Autodesk Inventor part; units mm, degrees
ref_plane "YZ Plane" through (0, 0, 0) normal (1, 0, 0) x (0, 1, 0)
ref_plane "XZ Plane" through (0, 0, 0) normal (0, 1, 0) x (-1, 0, 0)
ref_plane "XY Plane" through (0, 0, 0) normal (0, 0, 1) x (1, 0, 0)
sketch "Sketch1" plane through (0, 0, 0) normal (0, 1, 0) x (-1, 0, 0)
  line L0 (0, 0) -> (50, 0)
  line L1 (50, 0) -> (50, 48)
  line L2 (50, 48) -> (0, 48)
  line L3 (0, 48) -> (0, 0)
  dimension "d0" = 50
  dimension "d1" = 48
extrude "Extrusion1" add sketch "Sketch1" along normal blind 1.8
sketch "Sketch4" plane through (0, 1.8, 0) normal (0, 1, 0) x (1, 0, 0)
  line L0 (0, 0) -> (-50, 0)
  line L1 (-50, 0) -> (-50, -48)
  line L2 (-48, -17.9) -> (-40, -17.9)
  line L3 (-40, -17.9) -> (-40, -31.1)
  line L4 (-40, -31.1) -> (-48, -31.1)
  line L5 (-48, -31.1) -> (-48, -17.9)
  line L6 (-44, -24.5) -> (-44, -17.9)
  line L7 (-44, -24.5) -> (-40, -24.5)
  line L8 (-44, -24.5) -> (-44, -31.1)
  line L9 (-44, -24.5) -> (-48, -24.5)
  line L10 (-39, -17.9) -> (-31, -17.9)
  line L11 (-31, -17.9) -> (-31, -31.1)
  line L12 (-31, -31.1) -> (-39, -31.1)
  line L13 (-39, -31.1) -> (-39, -17.9)
  line L14 (-35, -24.5) -> (-35, -17.9)
  line L15 (-35, -24.5) -> (-31, -24.5)
  line L16 (-35, -24.5) -> (-35, -31.1)
  line L17 (-35, -24.5) -> (-39, -24.5)
  line L18 (-19, -17.9) -> (-11, -17.9)
  line L19 (-11, -17.9) -> (-11, -31.1)
  line L20 (-11, -31.1) -> (-19, -31.1)
  line L21 (-19, -31.1) -> (-19, -17.9)
  line L22 (-15, -24.5) -> (-15, -17.9)
  line L23 (-15, -24.5) -> (-11, -24.5)
  line L24 (-15, -24.5) -> (-15, -31.1)
  line L25 (-15, -24.5) -> (-19, -24.5)
  line L26 (-2, -17.9) -> (-2, -31.1)
  line L27 (-6, -24.5) -> (-6, -17.9)
  line L28 (-6, -24.5) -> (-2, -24.5)
  line L29 (-6, -24.5) -> (-6, -31.1)
  line L30 (-2, -31.1) -> (-10, -31.1)
  line L31 (-10, -17.9) -> (-2, -17.9)
  line L32 (-6, -24.5) -> (-10, -24.5)
  line L33 (-10, -31.1) -> (-10, -17.9)
  dimension "d4" = 8
  dimension "d6" = 13.2
  dimension "d7" = 24.5
  dimension "d8" = 6
  dimension "d9" = 8
  dimension "d10" = 13.2
  dimension "d12" = 9
  dimension "d13" = 8
  dimension "d14" = 13.2
  dimension "d15" = 8
  dimension "d16" = 13.2
  dimension "d17" = 20
  dimension "d18" = 9
extrude "Extrusion2" add sketch "Sketch4" along normal blind 10
sketch "Sketch5" plane through (0, 11.8, 0) normal (0, 1, 0) x (1, 0, 0)
  line L0 (-31, -31.1) -> (-31, -17.9)
  line L1 (-31, -17.9) -> (-39, -17.9)
  line L2 (-39, -17.9) -> (-39, -31.1)
  line L3 (-39, -31.1) -> (-31, -31.1)
  line L4 (-11, -31.1) -> (-11, -17.9)
  line L5 (-11, -17.9) -> (-19, -17.9)
  line L6 (-19, -17.9) -> (-19, -31.1)
  line L7 (-19, -31.1) -> (-11, -31.1)
  line L8 (-2, -17.9) -> (-10, -17.9)
  line L9 (-10, -17.9) -> (-10, -31.1)
  line L10 (-10, -31.1) -> (-2, -31.1)
  line L11 (-2, -31.1) -> (-2, -17.9)
  circle A0 centre (-44, -24.5) radius 3
  circle A1 centre (-35, -24.5) radius 3
  circle A2 centre (-15, -24.5) radius 3
  circle A3 centre (-6, -24.5) radius 3
  point P0 (0, 0)
  dimension "d21" = 6
  dimension "d23" = 6
  dimension "d24" = 6
  dimension "d25" = 6
extrude "Extrusion3" add sketch "Sketch5" along normal blind 9 contours A0 | A1 | A2 | A3
sketch "Sketch6" plane through (0, 0, 0) normal (0, -1, 0) x (1, 0, 0)
  line L0 (0, 0) -> (-50, 0)
  line L1 (0, 48) -> (0, 0)
  line L2 (-50, 48) -> (0, 48)
  line L3 (-50, 0) -> (-50, 48)
  line L4 (-0.1, 47.9) -> (-0.1, 0.1)
  line L5 (-0.1, 0.1) -> (-49.9, 0.1)
  line L6 (-49.9, 0.1) -> (-49.9, 47.9)
  line L7 (-49.9, 47.9) -> (-0.1, 47.9)
  dimension "d28" = 0.1
extrude "Extrusion4" add sketch "Sketch6" along normal blind 14 contours L4 L5 L6 L7
properties part number "ccpdu"
Here's how the part is built. I have some questions about the finished solid (model axes, mm). A direction names the side the tool comes from. Give positions to 0.01 mm unless a question says otherwise; leave off trailing zeros. Order: outer loops, then holes, each group sorted by start corner. A loop starts at its lowest first (then second) coordinate and runs counter-clockwise, first axis right, second up. Notation, with made-up numbers: M -20,73.5 L 37,73.5 A3 ccw 37,77.5 Z; hole C -8,62.25 d10. An arc over 180 degrees is marked long. Use a Markdown table: item, result. Add a question column.
1. I need wall thicknesses on probe 1 along X at (y, z) = (6, 24.5); probe 2 along X at (y, z) = (17, 23.5); probe 3 along Y at (x, z) = (-27.5, 41). Which ranges of each line are inside material? Lowest first, please. Write a range as from..to.
2. If we mould it in two halves opening along X, with no side actions, what happens to faces 1 (the flat face through (-25, -14, 24)), 2 (the flat face through (-31, 7, 24)), 3 (the flat face through (-50, 1, 24))? For each: +X half, -X half, draft (parallel to the pull), parting line (faces both ways), or undercut.
3. For pin 1 Ø11 at (y, z) = (-7, 19.5) entering from +X; pin 2 Ø8 at (y, z) = (7.5, 26.5) entering from -X; pin 3 Ø12 at (y, z) = (12, 6) entering from -X; pin 4 Ø4 at (x, z) = (-13, 15.5) entering from +Y, each with a flat end and sliding along its axis, tell me the tip position at first contact or that it passes through.
4. Suppose I cut it at A-A (y = 17). List the corners of the cut face in (x, z) for me, and give its area (3 significant figures).
5. On a 3-axis mill with a long thin cutter (end or side, diameter ignored), from which of +Z, -Z, +X, -X, +Y, -Y can I reach the whole of each face in a straight line? I mean faces 4 (the flat face through (-44, 7, 31.1)), 5 (the cylindrical face through (-3.23, 16.24, 23.35)), 6 (the flat face through (-19, 7, 25)). Say none if no direction works.
6. Suppose I cut it at B-B (x = -15). List the corners of the cut face in (y, z) for me.
Results list:
| question | item | result |
|---|---|---|
| 1 | probe 1 | x = -48..-40, -39..-31, -19..-11, -10..-2 |
| 1 | probe 2 | x = -46.83..-41.17, -37.83..-32.17, -17.83..-12.17, -8.83..-3.17 |
| 1 | probe 3 | y = -14..1.8 |
| 2 | face 1 | draft |
| 2 | face 2 | undercut |
| 2 | face 3 | -X half |
| 3 | pin 1 | stops at x = -0.1 |
| 3 | pin 2 | stops at x = -48 |
| 3 | pin 3 | passes through |
| 3 | pin 4 | stops at y = 1.8 |
| 4 | outline | C -44,24.5 d6; C -35,24.5 d6; C -15,24.5 d6; C -6,24.5 d6 |
| 4 | area | 113 mm² |
| 5 | face 4 | +Z, +X, -X, +Y |
| 5 | face 5 | +Y |
| 5 | face 6 | +Z, -Z, +Y |
| 6 | outline | M -14,0.1 L 0,0.1 L 0,0 L 1.8,0 L 1.8,17.9 L 11.8,17.9 L 11.8,21.5 L 20.8,21.5 L 20.8,27.5 L 11.8,27.5 L 11.8,31.1 L 1.8,31.1 L 1.8,48 L 0,48 L 0,47.9 L -14,47.9 Z |
